Geometry check sheet. Reference: the model listing, model coordinates, mm. A direction names the side the tool comes from. Round coordinates to 2 decimals unless told otherwise and drop trailing zeros. Write each loop counter-clockwise with the first axis right and the second up, starting at its lowest first coordinate (ties: lowest second). Pieces come first, ordered by that corner, then holes. Notation, with made-up numbers: (-26, -28) -> (-1, -28) arc R27 cw to (-1, 9) -> close; hole circle Ø10 at (-23.75, 79). An arc over 180 degrees is marked (long way). One line per question, with ' | ' between items.
```python
from build123d import *

# Parameters (mm, degrees)
F0_W      = 40
F0_H      = 40
F1_DEPTH  = 60
F2_W      = 10
F2_H      = 10
F3_DEPTH  = 50
F4_W      = 9.863964282
F4_H      = 30.0770029426
F5_DEPTH  = 20
F7_DEPTH  = 10
F8_DEPTH  = 30.001
F9_DEPTH  = 20.001
F10_W     = 30.136035718
F10_H     = 30
F11_DEPTH = 20
F12_DEPTH = 20


with BuildPart() as f1:
    # F0 (on Front) → F1 (new body)
    with BuildSketch(Plane.XZ):
        with Locations((20, 20)):
            Rectangle(F0_W, F0_H)
    extrude(amount=F1_DEPTH)

    # F2 (on face) → F3 (cut)
    with BuildSketch(Plane.XZ.offset(60)):
        with Locations((5, 5)):
            Rectangle(F2_W, F2_H)
    extrude(amount=-F3_DEPTH, mode=Mode.SUBTRACT)

    # F4 (on face) → F5 (cut)
    with BuildSketch(Plane.XY.offset(40)):
        with Locations((4.931982141, -15.0385014713)):
            Rectangle(F4_W, F4_H)
    extrude(amount=-F5_DEPTH, mode=Mode.SUBTRACT)

    # F6 (on face) → F7 (cut)
    with BuildSketch(Plane.XY.offset(40)):
        Polygon((0, -30.0770029426), (0, -60), (30.0770048052, -60), (30.0770048052, -30.0770029426), (9.863964282, -30.0770029426), align=None)
    extrude(amount=-F7_DEPTH, mode=Mode.SUBTRACT)

    # F8 (cut, through all): a face of the model
    f8_faces = [f1.faces().sort_by_distance(p)[0] for p in [
        (10, -35, 5),
    ]]
    extrude(f8_faces, amount=-F8_DEPTH, mode=Mode.SUBTRACT)

    # F9 (cut, through all): a face of the model
    f9_faces = [f1.faces().sort_by_distance(p)[0] for p in [
        (4.931982141, -15.0385014713, 20),
    ]]
    extrude(f9_faces, amount=-F9_DEPTH, mode=Mode.SUBTRACT)

    # F10 (on face) → F11 (cut)
    with BuildSketch(Plane.XY.offset(40)):
        with Locations((24.931982141, -15)):
            Rectangle(F10_W, F10_H)
    extrude(amount=-F11_DEPTH, mode=Mode.SUBTRACT)

    # F12 (cut): a face of the model
    f12_faces = [f1.faces().sort_by_distance(p)[0] for p in [
        (19.9704845436, -30.0770029426, 35),
    ]]
    extrude(f12_faces, amount=-F12_DEPTH, mode=Mode.SUBTRACT)


solid = f1.part
```
(1) Sectioned sample at D-D on z = 21.5. Record the cut outline in (x, y).
Resolved:
outline: (0, -60) -> (40, -60) -> (40, -30) -> (9.86, -30) -> (9.86, -30.08) -> (0, -30.08) -> close
(2) Sectioned sample at A-A on x = 23. Record the cut outline in (y, z), then the cut area to 3 significant figures.
Resolved:
outline: (-60, 10) -> (-10, 10) -> (-10, 0) -> (0, 0) -> (0, 20) -> (-30, 20) -> (-30, 30) -> (-60, 30) -> close | area: 1,000 mm2
(3) Sectioned sample at C-C on y = -36. Record the cut outline in (x, z).
Resolved:
outline: (0, 10) -> (40, 10) -> (40, 40) -> (30.08, 40) -> (30.08, 30) -> (0, 30) -> close
(4) Go/stop test with flat-tipped pins: pin 1 (9 mm diameter, centred on y = -21, z = 18.5, fed in from -X); pin 2 (22 mm diameter, centred on x = 27.5, z = 26, fed in from +Y); pin 3 (5 mm diameter, centred on y = -45.5, z = 35.5, fed in from -X); pin 4 (11 mm diameter, centred on x = 32.5, z = 3, fed in from -Y). Record where each tip stops, or that it passes through.
Resolved:
pin 1: stops at x = 9.86 | pin 2: stops at y = 0 | pin 3: stops at x = 30.08 | pin 4: stops at y = -10
(5) Sectioned sample at B-B on z = 31. Record the cut outline in (x, y), then the cut area to 3 significant figures.
Resolved:
outline: (30.08, -60) -> (40, -60) -> (40, -30) -> (30.08, -30) -> close | area: 298 mm2
(6) Material ranges on line 1 (Z direction, x = 10.5, y = -9); line 2 (X direction, y = -3, z = 15.5); line 3 (Y direction, x = 23, z = 7.5), recorded low to high.
Resolved:
line 1: z = 0 to 20 | line 2: x = 9.86 to 40 | line 3: y = -10 to 0
(7) Access from +Z, -Z, +X, -X, +Y, -Y to the whole of each face (thin tool, end or side, straight path). Record for faces 1 (the flat face through (25, -15, 20)), 2 (the flat face through (30.077, -45, 35)), 3 (the flat face through (25, -10, 5)).
Resolved:
face 1: +Z, +X, -X, +Y | face 2: +Z, -X, +Y, -Y | face 3: -Z, +X, -X, -Y
